Input: part model. Units: mm. Frame: model coordinates. Face numbers are marked on the shaded views. Round coordinates to 2 decimals unless told otherwise and drop trailing zeros. Order: outer loops, then holes, each group sorted by start corner. A loop starts at its lowest first (then second) coordinate and runs counter-clockwise, first axis right, second up. Notation, with made-up numbers: (50.25, 51.5) -> (91.25, 51.5) arc R27 ccw to (91.25, 87.5) -> close; hole circle Ø1 at (-28.75, 9.5). An arc over 180 degrees is marked (long way). Use a Markdown table: item, result.
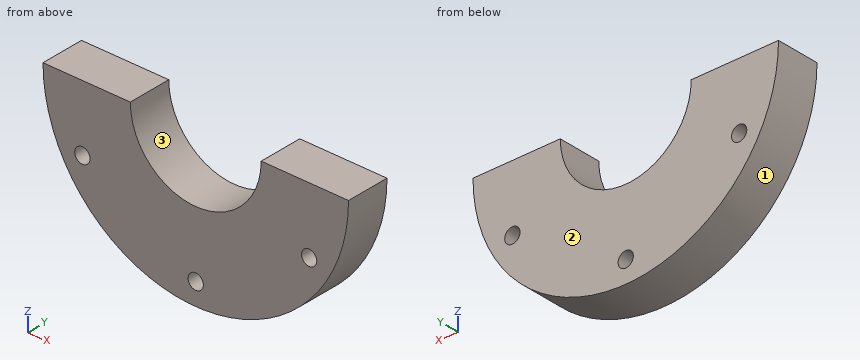
from build123d import *

# Parameters (mm, degrees)
F0_R     = 3.5
F1_DEPTH = 20


with BuildPart() as f1:
    # F0 (on Front) → F1 (new body)
    with BuildSketch(Plane.XZ):
        with BuildLine():
            ThreePointArc((-70, 0), (0, -70), (70, 0))
            Line((70, 0), (30, 0))
            ThreePointArc((30, 0), (0, -30), (-30, 0))
            Line((-30, 0), (-70, 0))
        make_face()
        with Locations((0, -60)):
            Circle(F0_R, mode=Mode.SUBTRACT)
        with Locations((-51.961524, -30)):
            Circle(F0_R, mode=Mode.SUBTRACT)
        with Locations((51.961524, -30)):
            Circle(F0_R, mode=Mode.SUBTRACT)
    extrude(amount=F1_DEPTH)


solid = f1.part
1) Pull-direction query (X, two-part tool) for the marked faces 1, 2 and 3; classes: +X half, -X half, draft (parallel to the pull), parting line (faces both ways), or undercut.
Results found:
| item | result |
|---|---|
| face 1 | parting line |
| face 2 | draft |
| face 3 | undercut |
2) Pin query (flat end, axial travel): pin 1 Ø4 at (x, z) = (51.96, -30) entering from +Y; pin 2 Ø3 at (x, y) = (42.5, -16) entering from -Z; pin 3 Ø9 at (x, z) = (-51.96, -30) entering from -Y; pin 4 Ø4 at (y, z) = (-6, -58.5) entering from -X. Return the tip coordinate at first contact, or that it passes through.
Results found:
| item | result |
|---|---|
| pin 1 | passes through |
| pin 2 | stops at z = -56.74 |
| pin 3 | stops at y = -20 |
| pin 4 | stops at x = -41.32 |
3) Cut plane C-C on z = -60. Return loops of the section in (x, y).
Results found:
| item | result |
|---|---|
| outline | (-36.06, -20) -> (-3.5, -20) -> (-3.5, 0) -> (-36.06, 0) -> close; (3.5, -20) -> (36.06, -20) -> (36.06, 0) -> (3.5, 0) -> close |
4) Line query: L1, parallel to Z at x = 0, y = -12.5; L2, parallel to X at y = -7, z = -12.5; L3, parallel to X at y = -1.75, z = -32. Output: solid intervals per line, ascending. Write a range as [from, to].
Results found:
| item | result |
|---|---|
| L1 | z = [-70, -63.5], [-56.5, -30] |
| L2 | x = [-68.87, -27.27], [27.27, 68.87] |
| L3 | x = [-62.26, -54.83], [-49.09, 49.09], [54.83, 62.26] |
5) Cut plane D-D on x = 16. Return loops of the section in (y, z), and give its area (3 significant figures).
Results found:
| item | result |
|---|---|
| outline | (-20, -68.15) -> (0, -68.15) -> (0, -25.38) -> (-20, -25.38) -> close |
| area | 855 mm² |
6) Cut plane B-B on y = -13.25. Return loops of the section in (x, z).
Results found:
| item | result |
|---|---|
| outline | (-70, 0) arc R70 ccw to (70, 0) -> (30, 0) arc R30 cw to (-30, 0) -> close; hole circle Ø7 at (-51.96, -30); hole circle Ø7 at (0, -60); hole circle Ø7 at (51.96, -30) |
7) Cut plane A-A on x = 0. Return loops of the section in (y, z), and give its area (3 significant figures).
Results found:
| item | result |
|---|---|
| outline | (-20, -70) -> (0, -70) -> (0, -63.5) -> (-20, -63.5) -> close; (-20, -56.5) -> (0, -56.5) -> (0, -30) -> (-20, -30) -> close |
| area | 660 mm² |
